Could you check a few things on this drawing? It's one solid part, dimensions in mm from its lowest x, y, z. A direction names the side the tool comes from. Round coordinates to 2 decimals unless told otherwise and drop trailing zeros. Loops run counter-clockwise (first coordinate to the right, second up) from the corner with the lowest first, then second, coordinate; pieces in that order, holes last. Notation, with made-up numbers: M -26.5,16 L 22.5,16 A24 ccw 22.5,43 Z; hole C 51,64 d2. An arc over 180 degrees is marked long. Return JSON: item names as keys, results as strings.
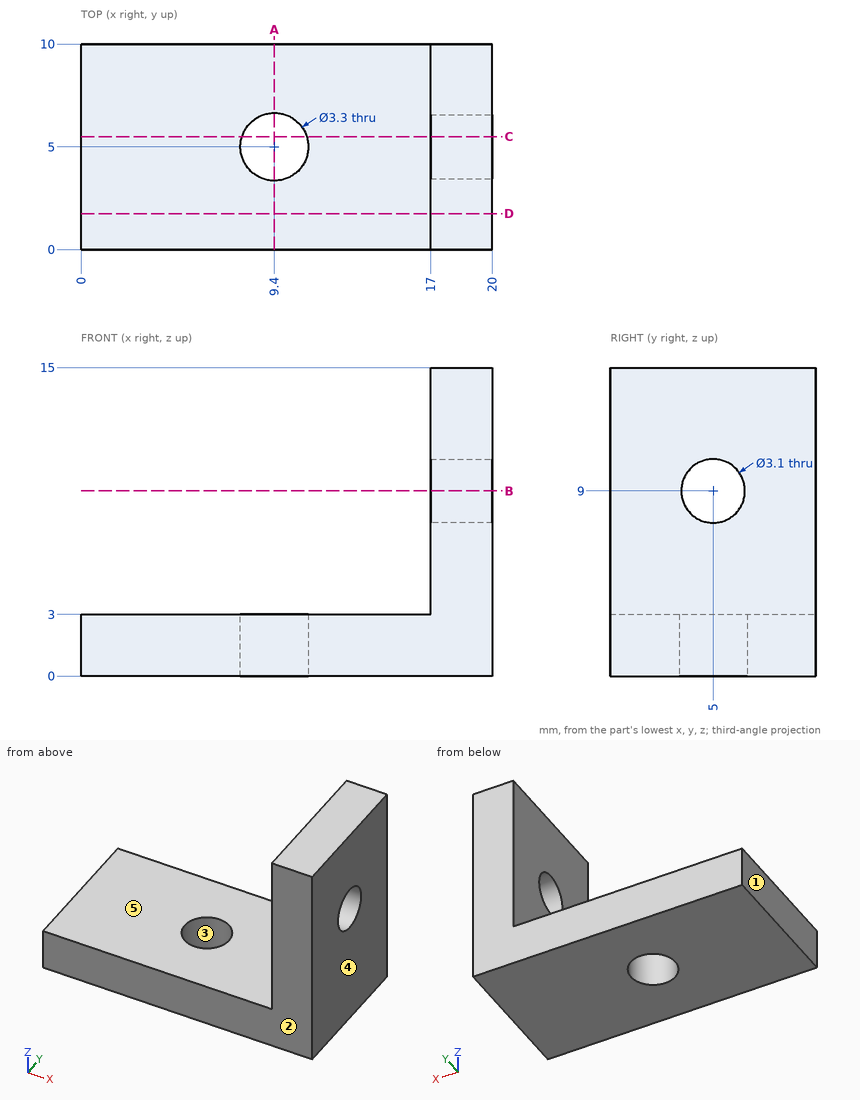
Q1. Suppose I cut it at D-D, the plane y = 1.75. Please give me the cut outline in (x, z), plus the area to 3 significant figures.
Results:
{"outline": "M 0,0 L 20,0 L 20,15 L 17,15 L 17,3 L 0,3 Z", "area": "96.0 mm2"}
Q2. On a 3-axis mill with a long thin cutter (end or side, diameter ignored), from which of +Z, -Z, +X, -X, +Y, -Y can I reach the whole of each face in a straight line? I mean the marked faces 4 and 5. Say none if no direction works.
Results:
{"face 4": "+Z, -Z, +X, +Y, -Y", "face 5": "+Z, -X, +Y, -Y"}
Q3. I'm going to push flat-ended pins straight in: pin 1 Ø2.5 at (x, y) = (9.4, 5) entering from -Z; pin 2 Ø4 at (y, z) = (2, 8.5) entering from -X. Where does each tip first touch, or does it pass through?
Results:
{"pin 1": "passes through", "pin 2": "stops at x = 17"}
Q4. Thinking about a two-plate mould opening in Y: for the marked faces 1, 2 and 3, which applies, pulls with the +Y half, pulls with the -Y half, needs draft (parallel to the pull), parting line crosses it, or undercut?
Results:
{"face 1": "needs draft", "face 2": "pulls with the -Y half", "face 3": "undercut"}
Q5. If I drill on line 1 along Y through (x, z) = (9.4, 1.05); line 2 along Y through (x, z) = (17.85, 9); line 3 along X through (y, z) = (6.75, 13.75), over which ranges is the centre line in solid material (lowest first)?
Results:
{"line 1": "y = 0 to 3.35, 6.65 to 10", "line 2": "y = 0 to 3.45, 6.55 to 10", "line 3": "x = 17 to 20"}
Q6. Suppose I cut it at C-C, the plane y = 5.5. Please give me the cut outline in (x, z).
Results:
{"outline": "M 0,0 L 7.83,0 L 7.83,3 L 0,3 Z; M 10.97,0 L 20,0 L 20,7.53 L 17,7.53 L 17,3 L 10.97,3 Z; M 17,10.47 L 20,10.47 L 20,15 L 17,15 Z"}
Q7. Suppose I cut it at B-B, the plane z = 9. Please give me the cut outline in (x, y), plus the area to 3 significant figures.
Results:
{"outline": "M 17,0 L 20,0 L 20,3.45 L 17,3.45 Z; M 17,6.55 L 20,6.55 L 20,10 L 17,10 Z", "area": "20.7 mm2"}
Q8. Suppose I cut it at A-A, the plane x = 9.4. Please give me the cut outline in (y, z).
Results:
{"outline": "M 0,0 L 3.35,0 L 3.35,3 L 0,3 Z; M 6.65,0 L 10,0 L 10,3 L 6.65,3 Z"}
